Study the drawing (mm; zero at the part's minimum x, y, z) and answer. A direction names the side the tool comes from. Round coordinates to 2 decimals unless told otherwise and drop trailing zeros. Write each loop counter-clockwise with the first axis right and the second up, starting at its lowest first coordinate (ties: lowest second). Pieces come first, ordered by that corner, then holes. Notation, with made-up numbers: (50.5, 76.25) - (82.5, 76.25) arc R26 cw to (82.5, 108.25) - close; hole circle Ø4 at (40, -10.5). An arc over 180 degrees is marked (long way). Use one line per item in the form item = value. Start each with the question number.
1) The part is cut by section A-A, the plane z = 7.75. Give the vertices of the cut face in (x, y) (3 decimals), plus the area to 3 significant figures.
2) The part is cut by section B-B, the plane z = 1.75. Give the vertices of the cut face in (x, y) (3 decimals).
3) For the marked faces 4 and 5, determine the directions among +Z, -Z, +X, -X, +Y, -Y from which every point of the face is accessible in a straight line to the end or side of a thin tool.
4) Each of these flat-tipped pins is pushed along its axis until it touches: pin 1 (4 mm diameter, centred on y = 20.5, z = 6.5, fed in from +X); pin 2 (3 mm diameter, centred on y = 13, z = 3, fed in from +X); pin 3 (6 mm diameter, centred on y = 21, z = 6.5, fed in from +X); pin 4 (1 mm diameter, centred on x = 13.5, z = 4, fed in from -Y). Where does it stop, or does it pass through?
5) For a pull along X with two mould halves and no side action, classify the marked faces 1, 2 and 3 as released by +X, released by -X, zero draft, split by the parting line, or undercut.
6) Consider line 1 along X through (y, z) = (12, 6.5); line 2 along Y through (x, z) = (7.5, 4.25); line 3 along Y through (x, z) = (6, 1.5). Determine where each line is inside the solid, lowest interval first. Write a range as from..to.
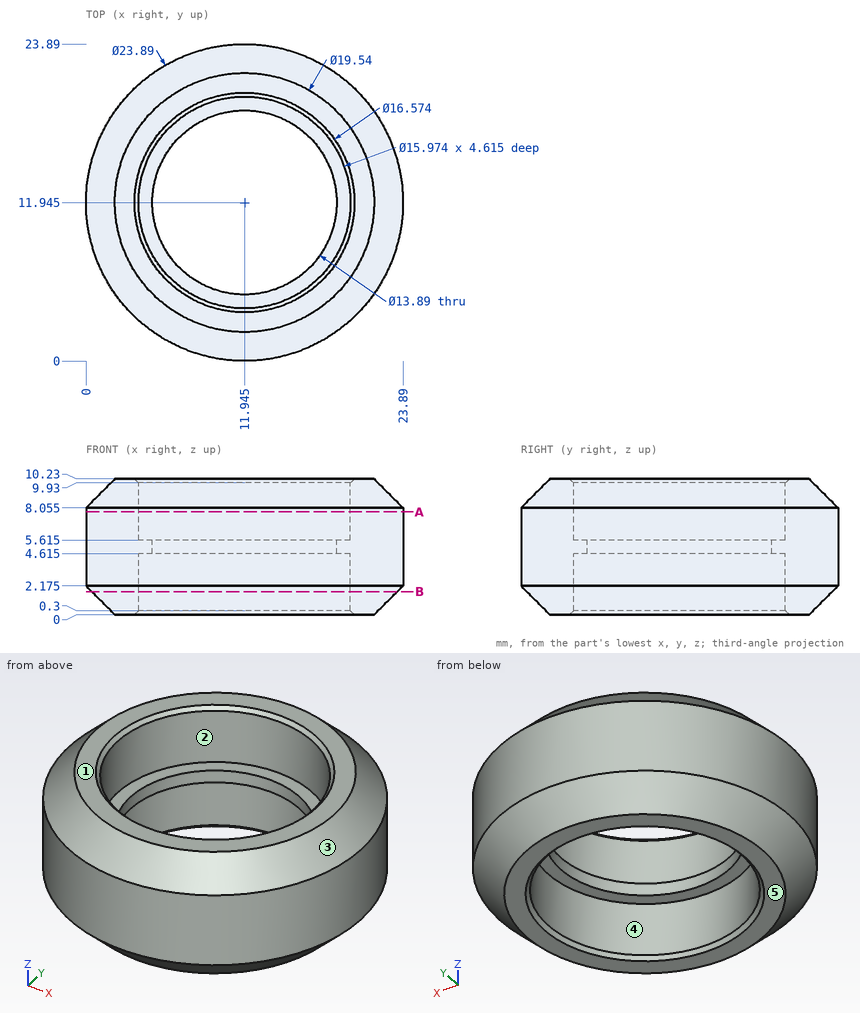
Geometry results:
q1.outline = circle Ø23.89 at (11.945, 11.945); hole circle Ø15.974 at (11.945, 11.945)
q1.area = 248 mm2
q2.outline = circle Ø23.04 at (11.945, 11.945); hole circle Ø15.974 at (11.945, 11.945)
q3.face_4 = -Z
q3.face_5 = -Z, +X, -X, +Y, -Y
q4.pin_1 = 21.93
q4.pin_2 = 23.89
q4.pin_3 = 22.24
q4.pin_4 = 0.05
q5.face_1 = zero draft
q5.face_2 = undercut
q5.face_3 = split by the parting line
q6.line_1 = 0..3.96, 19.93..23.89
q6.line_2 = 0.86..5.31, 18.58..23.03
q6.line_3 = 2.37..6.61, 17.28..21.52
